```python
from build123d import *

# Parameters (mm, degrees)
BOSS_EXTRUDE1_DEPTH = 6
SKETCH2_R           = 2
SKETCH2_R_2         = 1.6
CUT_EXTRUDE1_DEPTH  = 7
CHAMFER1_SIZE       = 0.5
CUT_EXTRUDE2_DEPTH  = 7
SKETCH5_R           = 1.6
CUT_EXTRUDE3_DEPTH  = 7


with BuildPart() as part:
    # Sketch1 → Boss-Extrude1 (new body)
    with BuildSketch(Plane.XY):
        with BuildLine():
            Line((-7.5, 20), (-66, 20))
            Line((-66, 20), (-66, 26))
            Line((-66, 26), (-82, 26))
            Line((-82, 26), (-82, 20))
            Line((-82, 20), (-86, 20))
            Line((-86, 20), (-86, 13))
            Line((-86, 13), (-64, 13))
            ThreePointArc((-64, 13), (-60.433883594, 11.825226811), (-58.264226502, 8.760937927))
            Line((-58.264226502, 8.760937927), (-50.735773498, -15.760937927))
            ThreePointArc((-50.735773498, -15.760937927), (-48.566116406, -18.825226811), (-45, -20))
            Line((-45, -20), (-35.321388767, -20))
            ThreePointArc((-35.321388767, -20), (0, -10.5), (35.321388767, -20))
            Line((35.321388767, -20), (45, -20))
            ThreePointArc((45, -20), (48.566116406, -18.825226811), (50.735773498, -15.760937927))
            Line((50.735773498, -15.760937927), (58.264226502, 8.760937927))
            ThreePointArc((58.264226502, 8.760937927), (60.433883594, 11.825226811), (64, 13))
            Line((64, 13), (86, 13))
            Line((86, 13), (86, 20))
            Line((86, 20), (82, 20))
            Line((82, 20), (82, 26))
            Line((82, 26), (66, 26))
            Line((66, 26), (66, 20))
            Line((66, 20), (7.5, 20))
            Line((7.5, 20), (7.5, 26))
            Line((7.5, 26), (3, 26))
            Line((3, 26), (3, 8))
            Line((3, 8), (-3, 8))
            Line((-3, 8), (-3, 26))
            Line((-3, 26), (-7.5, 26))
            Line((-7.5, 26), (-7.5, 20))
        make_face()
    extrude(amount=BOSS_EXTRUDE1_DEPTH)

    # Sketch2 → Cut-Extrude1 (cut, through all)
    with BuildSketch(Plane.XY.offset(6)):
        with Locations((39, -13)):
            Circle(SKETCH2_R)
        with Locations((39, 13)):
            Circle(SKETCH2_R)
        with Locations((25, -3.2)):
            Circle(SKETCH2_R_2)
        with Locations((-25, -3.2)):
            Circle(SKETCH2_R_2)
    cut_extrude1 = extrude(amount=-CUT_EXTRUDE1_DEPTH, mode=Mode.SUBTRACT)

    # Mirror1: Cut-Extrude1 across plane
    add(cut_extrude1.mirror(Plane(origin=(0, 0, 0), x_dir=(0, 0, 1), z_dir=(1, 0, 0))), mode=Mode.SUBTRACT)

    # Chamfer1
    chamfer1_edges = [part.edges().sort_by_distance(p)[0] for p in [
        (66, 26, 3),
        (82, 26, 3),
        (-82, 26, 3),
        (-66, 26, 3),
    ]]
    chamfer(chamfer1_edges, length=CHAMFER1_SIZE)

    # Sketch4 → Cut-Extrude2 (cut, through all)
    with BuildSketch(Plane.XY.offset(6)):
        Polygon((-29.48, 20), (-29.48, 15), (-31.45, 15), (-31.45, 14.5), (-30.7, 14.5), (-30.7, 12), (-29.48, 12), (-29.48, 9), (-26.52, 9), (-26.52, 12), (-25.3, 12), (-25.3, 14.5), (-24.55, 14.5), (-24.55, 15), (-26.52, 15), (-26.52, 20), align=None)
        Polygon((26.52, 20), (26.52, 15), (24.55, 15), (24.55, 14.5), (25.3, 14.5), (25.3, 12), (26.52, 12), (26.52, 9), (29.48, 9), (29.48, 12), (30.7, 12), (30.7, 14.5), (31.45, 14.5), (31.45, 15), (29.48, 15), (29.48, 20), align=None)
    extrude(amount=-CUT_EXTRUDE2_DEPTH, mode=Mode.SUBTRACT)

    # Sketch5 → Cut-Extrude3 (cut, through all)
    with BuildSketch(Plane.XY.offset(6)):
        with Locations((-15, -2.2)):
            Circle(SKETCH5_R)
    extrude(amount=-CUT_EXTRUDE3_DEPTH, mode=Mode.SUBTRACT)


solid = part.part
```
Source: CAD feature listing. Evaluate the final solid. Frame: model axes, mm. A direction names the side the tool comes from. Round coordinates to 2 decimals unless told otherwise and drop trailing zeros. Order: outer loops, then holes, each group sorted by start corner. A loop starts at its lowest first (then second) coordinate and runs counter-clockwise, first axis right, second up. Notation, with made-up numbers: (52, -2.5) -> (107, -2.5) arc R15 ccw to (107, 2.5) -> close; hole circle Ø7 at (-4, 29). An arc over 180 degrees is marked (long way). Use CSV: the item, a comma, the result in double quotes.
(1) Pull-direction query (X, two-part tool) for faces 1 (the face through (-37.526, -11.648, 3.042)), 2 (the face through (-48.6, -18.8, 3)), 3 (the face through (29.48, 17, 3)), 4 (the face through (-75, 13, 3)); classes: +X half, -X half, draft (parallel to the pull), parting line (faces both ways), or undercut.
Report:
face 1,"undercut"
face 2,"-X half"
face 3,"undercut"
face 4,"draft"
(2) Section D-D on z = 3.4. Count the separate pieces of the cut face and the enclosed holes in it, and give its area (3 significant figures).
Report:
separate pieces,"1"
enclosed holes,"7"
area,"4,370 mm^2"
(3) First-contact query: pin 1 Ø3.5 at (x, y) = (-39, -13) entering from +Z; pin 2 Ø0.8 at (x, z) = (-31, 4.5) entering from +Y; pin 3 Ø1.5 at (y, z) = (-3.5, 2) entering from +X; pin 4 Ø3 at (y, z) = (10, 2) entering from +X. Flat tips, straight axial feed; report the tip coordinate or a pass-through.
Report:
pin 1,"through"
pin 2,"y = 20"
pin 3,"x = 54.73"
pin 4,"x = 60.03"
(4) Section B-B on x = 39. Return the cut outline in (y, z), and give its area (3 significant figures).
Report:
outline,"(-20, 0) -> (-15, 0) -> (-15, 6) -> (-20, 6) -> close; (-11, 0) -> (11, 0) -> (11, 6) -> (-11, 6) -> close; (15, 0) -> (20, 0) -> (20, 6) -> (15, 6) -> close"
area,"192 mm^2"
(5) Access query for faces 5 (the face through (37.526, 14.352, 3.042)), 6 (the face through (84, 20, 3)), 7 (the face through (-66, 23, 3)). Directions: +Z, -Z, +X, -X, +Y, -Y. A direction counts if a zero-diameter tool reaches every point of the face in a straight line with its end or side. Return the directions, or none.
Report:
face 5,"+Z, -Z"
face 6,"+Z, -Z, +X, +Y"
face 7,"+Z, -Z, +Y"
(6) Section A-A on y = -13. Return the cut outline in (x, z).
Report:
outline,"(-51.58, 0) -> (-41, 0) -> (-41, 6) -> (-51.58, 6) -> close; (-37, 0) -> (-18.6, 0) -> (-18.6, 6) -> (-37, 6) -> close; (18.6, 0) -> (37, 0) -> (37, 6) -> (18.6, 6) -> close; (41, 0) -> (51.58, 0) -> (51.58, 6) -> (41, 6) -> close"
(7) Ray query, L1, parallel to X at y = 21.5, z = 4.9; L2, parallel to Y at x = -43, z = 3.35; L3, parallel to Y at x = 39.5, z = 1.4. Return the intervals inside material, ascending.
Report:
L1,"-82 to -66, -7.5 to -3, 3 to 7.5, 66 to 82"
L2,"-20 to 20"
L3,"-20 to -14.94, -11.06 to 11.06, 14.94 to 20"
(8) Section C-C on x = -72.5. Return the cut outline in (y, z).
Report:
outline,"(13, 0) -> (26, 0) -> (26, 6) -> (13, 6) -> close"
